from build123d import *

# Parameters (mm, degrees)
SKETCH1_W                 = 50.8
SKETCH1_H                 = 203.2
BOSS_EXTRUDE1_DEPTH       = 15.875
F_1_4_CLEARANCE_HOLE1_D   = 6.7564
SKETCH5_R                 = 6.35
CUT_EXTRUDE1_DEPTH        = 16.875
SKETCH6_R                 = 14.2875
CUT_EXTRUDE2_DEPTH        = 7.9375
F_4_40_TAPPED_HOLE1_D     = 2.2606
F_4_40_TAPPED_HOLE1_DEPTH = 7.62
F_4_40_TAPPED_HOLE1_TIP   = 0.679152758


with BuildPart() as part:
    # Sketch1 → Boss-Extrude1 (new body)
    with BuildSketch(Plane.XY):
        with Locations((0, 76.2)):
            Rectangle(SKETCH1_W, SKETCH1_H)
    extrude(amount=BOSS_EXTRUDE1_DEPTH)

    # 1/4 Clearance Hole1 (through all)
    with Locations(Plane.XY.offset(15.875)):
        with Locations((12.7, 0), (-12.7, 0)):
            Hole(F_1_4_CLEARANCE_HOLE1_D / 2)

    # Sketch5 → Cut-Extrude1 (cut, through all)
    with BuildSketch(Plane(origin=(0, 0, 0), x_dir=(-1, 0, 0), z_dir=(0, 0, -1))):
        with Locations((0, 158.75)):
            Circle(SKETCH5_R)
        with Locations((0, 76.2)):
            Circle(SKETCH5_R)
    extrude(amount=-CUT_EXTRUDE1_DEPTH, mode=Mode.SUBTRACT)

    # Sketch6 → Cut-Extrude2 (cut)
    with BuildSketch(Plane.XY.offset(15.875)):
        with Locations((0, 76.2)):
            Circle(SKETCH6_R)
    extrude(amount=-CUT_EXTRUDE2_DEPTH, mode=Mode.SUBTRACT)

    # #4-40 Tapped Hole1
    with Locations(Plane.XY.offset(15.875)):
        with Locations((0, 99.187), (0, 53.213)):
            Hole(F_4_40_TAPPED_HOLE1_D / 2, depth=F_4_40_TAPPED_HOLE1_DEPTH)
            with Locations((0, 0, -(F_4_40_TAPPED_HOLE1_DEPTH + F_4_40_TAPPED_HOLE1_TIP / 2))):  # 118° drill point
                Cone(0, F_4_40_TAPPED_HOLE1_D / 2, F_4_40_TAPPED_HOLE1_TIP, mode=Mode.SUBTRACT)


solid = part.part
Verification items for the finished model (mm, model axes). A direction names the side the tool comes from. Give positions to 0.01 mm unless a question says otherwise; leave off trailing zeros. Loops run counter-clockwise (first coordinate to the right, second up) from the corner with the lowest first, then second, coordinate; pieces in that order, holes last.
1) Sectioned sample at D-D, the plane y = 158.75. Enter the section's corners in (x, z) (3 decimals), then the cut area to 3 significant figures.
2) Thickness scan on line 1 along Y through (x, z) = (0, 12); line 2 along X through (y, z) = (158.5, 3.75); line 3 along Y through (x, z) = (4.5, 5.5). Record the ranges inside material, lowest first.
3) Depth check by flat-ended pin: pin 1 Ø8.5 at (x, y) = (5.5, 80) entering from +Z. Enter the tip coordinate at first touch or a pass-through.
4) Sectioned sample at B-B, the plane y = 0. Enter the section's corners in (x, z) (3 decimals).
5) Set-up check for faces 4 (the cylindrical face through (-1.86, 90.366, 11.962)), 5 (the cylindrical face through (1.38, 70, 3.91)): record each of +Z, -Z, +X, -X, +Y, -Y from which the full face is reachable in a straight line by a thin tool's end or side.
6) Sectioned sample at C-C, the plane z = 3. Enter the section's corners in (x, y).
7) Draft check along X on faces 1 (the flat face through (6, 73, 7.938)), 2 (the flat face through (-25.4, 75, 8)), 3 (the flat face through (0, 177.8, 8)). Enter one of: pulls with the +X half, pulls with the -X half, needs draft (parallel to the pull), parting line crosses it, or undercut.
Answers:
1. outline: (-25.4, 0) - (-6.35, 0) - (-6.35, 15.875) - (-25.4, 15.875) - close; (6.35, 0) - (25.4, 0) - (25.4, 15.875) - (6.35, 15.875) - close
1. area: 605 mm2
2. line 1: y = -25.4 to 52.08, 54.34 to 61.91, 90.49 to 98.06, 100.32 to 152.4, 165.1 to 177.8
2. line 2: x = -25.4 to -6.35, 6.35 to 25.4
2. line 3: y = -25.4 to 71.72, 80.68 to 154.27, 163.23 to 177.8
3. pin 1: stops at z = 7.94
4. outline: (-25.4, 0) - (-16.078, 0) - (-16.078, 15.875) - (-25.4, 15.875) - close; (-9.322, 0) - (9.322, 0) - (9.322, 15.875) - (-9.322, 15.875) - close; (16.078, 0) - (25.4, 0) - (25.4, 15.875) - (16.078, 15.875) - close
5. face 4: +Z
5. face 5: +Z, -Z
6. outline: (-25.4, -25.4) - (25.4, -25.4) - (25.4, 177.8) - (-25.4, 177.8) - close; hole circle Ø6.76 at (-12.7, 0); hole circle Ø12.7 at (0, 76.2); hole circle Ø12.7 at (0, 158.75); hole circle Ø6.76 at (12.7, 0)
7. face 1: undercut
7. face 2: pulls with the -X half
7. face 3: needs draft
